For this review, take the finished solid that the model builds, in its own axes (mm). A direction names the side the tool comes from. Round coordinates to 2 decimals unless told otherwise and drop trailing zeros. Loops run counter-clockwise (first coordinate to the right, second up) from the corner with the lowest first, then second, coordinate; pieces in that order, holes last.
```python
from build123d import *

# Parameters (mm, degrees)
EXTRUDE_1_DEPTH = 21
EXTRUDE_1_TAPER = 5
SKETCH_2_R      = 10
EXTRUDE_2_DEPTH = 8


with BuildPart() as part:
    # Эскиз1 → Бобышка-Вытянуть1 (new body)
    with BuildSketch(Plane.XY):
        with BuildLine():
            ThreePointArc((206.902825712, -28.037707575), (208.16042902, -13.627270923), (194.643197369, -8.47686326))
            Line((194.643197369, -8.47686326), (178.352602864, -13.211762774))
            ThreePointArc((178.352602864, -13.211762774), (164.281318134, -14.974601832), (150.3601632, -12.270882024))
            Line((150.3601632, -12.270882024), (21.714759937, 34.696764669))
            ThreePointArc((21.714759937, 34.696764669), (18.576858011, 34.793189635), (16, 33))
            ThreePointArc((16, 33), (8.94427191, 27.11145618), (0, 25))
            ThreePointArc((0, 25), (-24.017605322, 6.939354046), (-13.333333333, -21.147629234))
            ThreePointArc((-13.333333333, -21.147629234), (-5.735545873, -29.916516988), (-4.284649798, -41.428018512))
            ThreePointArc((-4.284649798, -41.428018512), (6.155658081, -59.36704661), (8.411759167, -80))
            Line((8.411759167, -80), (-6.939849245, -232.746575098))
            ThreePointArc((-6.939849245, -232.746575098), (0.139115456, -244.91798346), (13.910401615, -241.984282673))
            Line((13.910401615, -241.984282673), (206.902825712, -28.037707575))
        make_face()
    extrude(amount=EXTRUDE_1_DEPTH, taper=EXTRUDE_1_TAPER)

    # Эскиз2 → Бобышка-Вытянуть2 (add)
    with BuildSketch(Plane.XY.offset(21)):
        with Locations((5, -233.946575098)):
            Circle(SKETCH_2_R)
        with Locations((197.992424097, -20)):
            Circle(SKETCH_2_R)
    extrude(amount=EXTRUDE_2_DEPTH)


solid = part.part
```
(1) For faces 1 (the flat face through (65, -72, 0)), 2 (the cylindrical face through (2.8, -243.7, 24.9)), 3 (the flat face through (1.53, -157.53, 10.35)), 4 (the flat face through (111.08, -132.91, 10.35)), 5 (the flat face through (186.637, -11.747, 10.353)), list the 3-axis set-ups (+Z, -Z, +X, -X, +Y, -Y) from which the entire face can be reached by the end or side of a thin tool; tool diameter is ignored.
(2) For L1, parallel to Z at x = 66.5, y = -11; L2, parallel to Y at x = 104, z = 11.25; L3, parallel to Y at x = 111, z = 3, list the stretches that pass through material, from the lowest coordinate up.
(3) The part is to be moulded in two halves that separate along X. For faces 6 (the flat face through (5, -234, 29)), 7 (the conical face through (6.946, -58.793, 10.647)), 8 (the conical face through (164.453, -15.912, 10.647)), say which applies: pulls with the +X half, pulls with the -X half, needs draft (parallel to the pull), parting line crosses it, or undercut.
(4) Add section A-A (z = 14). Give the boundary of the cut face in (x, y).
(5) Add section B-B (y = -221). Give the boundary of the cut face in (x, z), plus the area to 3 significant figures.
(6) Insertion check: pin 1 Ø5 at (x, z) = (109.5, 11) entering from +Y; pin 2 Ø10 at (y, z) = (-158, 8.5) entering from -X; pin 3 Ø8 at (x, y) = (0, -109.5) entering from +Z; pin 4 Ø2 at (x, z) = (76, 5.5) entering from +Y. Each pin has a flat end and moves straight along its axis. Give the tip position at first contact, or say it passes through.
Outcome:
1. face 1: -Z, +X, -X, +Y, -Y
1. face 2: +Z
1. face 3: +Z, -X
1. face 4: +Z, +X, -Y
1. face 5: +Z, +Y
2. L1: z = 0 to 21
2. L2: y = -140.64 to 3.61
2. L3: y = -133.96 to 1.82
3. face 6: needs draft
3. face 7: pulls with the -X half
3. face 8: undercut
4. outline: (-12.68, -20.11) arc R21.22 cw to (-2.99, -41.04) arc R51.22 cw to (9.63, -80.12) - (-5.72, -232.87) arc R10.78 ccw to (13, -241.16) - (205.99, -27.22) arc R10.78 ccw to (194.99, -9.65) - (178.69, -14.39) arc R46.22 cw to (149.94, -13.42) - (21.29, 33.55) arc R3.78 ccw to (16.98, 32.27) arc R21.22 cw to (0, 23.78) arc R23.78 ccw to start
5. outline: (-5.76, 0) - (32.84, 0) - (30.37, 21) - (-3.91, 21) - close
5. area: 765 mm2
6. pin 1: stops at y = 2.56
6. pin 2: stops at x = 0.65
6. pin 3: passes through
6. pin 4: stops at y = 14.74
